Work out the finished part from the listing and answer in its coordinate system (mm). A direction names the side the tool comes from. Round coordinates to 2 decimals unless told otherwise and drop trailing zeros. Loops run counter-clockwise (first coordinate to the right, second up) from the corner with the lowest first, then second, coordinate; pieces in that order, holes last.
```python
from build123d import *

# Parameters (mm, degrees)
SKETCH1_W           = 122
SKETCH1_H           = 30
SKETCH1_R           = 2.2
BOSS_EXTRUDE1_DEPTH = 3
SKETCH2_W           = 46
SKETCH2_H           = 86.2
SKETCH2_R           = 1.75
BOSS_EXTRUDE2_DEPTH = 3
BOSS_EXTRUDE3_DEPTH = 3
FILLET1_R           = 10
CHAMFER1_SIZE       = 1.65
SKETCH4_W           = 32
SKETCH4_H           = 16
SKETCH4_R           = 2
BOSS_EXTRUDE4_DEPTH = 3
CHAMFER2_SIZE       = 6


with BuildPart() as part:
    # Sketch1 → Boss-Extrude1 (new body)
    with BuildSketch(Plane.XY):
        Rectangle(SKETCH1_W, SKETCH1_H)
        with Locations((-56, 5)):
            Circle(SKETCH1_R, mode=Mode.SUBTRACT)
        with Locations(Location((-56, -5, 0), (0, 0, 180))):
            Circle(SKETCH1_R, mode=Mode.SUBTRACT)
        with Locations((56, -5)):
            Circle(SKETCH1_R, mode=Mode.SUBTRACT)
        with Locations(Location((56, 5, 0), (0, 0, 180))):
            Circle(SKETCH1_R, mode=Mode.SUBTRACT)
    extrude(amount=BOSS_EXTRUDE1_DEPTH)

    # Sketch2 → Boss-Extrude2 (add)
    with BuildSketch(Plane.XY.offset(3)):
        with Locations((0, 58.1)):
            Rectangle(SKETCH2_W, SKETCH2_H)
        with Locations((0, 17.3)):
            Circle(SKETCH2_R, mode=Mode.SUBTRACT)
        with Locations((10, 54.9)):
            Circle(SKETCH2_R, mode=Mode.SUBTRACT)
        with Locations((0, 31.2)):
            Circle(SKETCH2_R, mode=Mode.SUBTRACT)
        with Locations(Location((-10, 54.9, 0), (0, 0, 180))):
            Circle(SKETCH2_R, mode=Mode.SUBTRACT)
    extrude(amount=-BOSS_EXTRUDE2_DEPTH)

    # Sketch3 → Boss-Extrude3 (add)
    with BuildSketch(Plane.XY.offset(3)):
        Polygon((-47, 15), (-23, 39), (-23, 15), align=None)
        Polygon((23, 39), (23, 15), (47, 15), align=None)
    extrude(amount=-BOSS_EXTRUDE3_DEPTH)

    # Fillet1
    fillet1_edges = [part.edges().sort_by_distance(p)[0] for p in [
        (-47, 15, 1.5),
        (-23, 39, 1.5),
        (23, 39, 1.5),
        (47, 15, 1.5),
    ]]
    fillet(fillet1_edges, radius=FILLET1_R)

    # Chamfer1
    chamfer1_edges = [part.edges().sort_by_distance(p)[0] for p in [
        (-1.75, 17.3, 3),
        (8.25, 54.9, 3),
        (-1.75, 31.2, 3),
        (-8.25, 54.9, 3),
    ]]
    chamfer(chamfer1_edges, length=CHAMFER1_SIZE)

    # Sketch4 → Boss-Extrude4 (add)
    with BuildSketch(Plane(origin=(23, 0, 0), x_dir=(0, 0, -1), z_dir=(1, 0, 0))):
        with Locations((13, 93.2)):
            Rectangle(SKETCH4_W, SKETCH4_H)
        with Locations(Location((23, 93.2, 0), (0, 0, 90))):
            Circle(SKETCH4_R, mode=Mode.SUBTRACT)
        with Locations(Location((6, 93.2, 0), (0, 0, 270))):
            Circle(SKETCH4_R, mode=Mode.SUBTRACT)
    boss_extrude4 = extrude(amount=-BOSS_EXTRUDE4_DEPTH)

    # Mirror1: Boss-Extrude4 across plane
    add(boss_extrude4.mirror(Plane(origin=(0, 0, 0), x_dir=(0, 0, 1), z_dir=(1, 0, 0))))

    # Chamfer2
    chamfer2_edges = [part.edges().sort_by_distance(p)[0] for p in [
        (21.5, 85.2, 0),
        (-21.5, 85.2, 0),
    ]]
    chamfer(chamfer2_edges, length=CHAMFER2_SIZE)


solid = part.part
```
1. Given pin 1 (1.5 mm diameter, centred on x = 21.5, z = -15.5, fed in from -Y); pin 2 (4 mm diameter, centred on x = -56, y = 5, fed in from -Z); pin 3 (6.5 mm diameter, centred on y = 87.5, z = -18.5, fed in from +X); pin 4 (1.5 mm diameter, centred on x = -54.5, z = 1, fed in from +Y), each flat-ended and moving along its own axis, determine where each tip first touches the part or whether it passes through.
Answer key:
pin 1: stops at y = 85.2
pin 2: passes through
pin 3: stops at x = 23
pin 4: stops at y = 15
2. Find section B-B (y = 31.2). Write down the section's boundary in (x, z).
Answer key:
outline: (-30.8, 0) - (-1.75, 0) - (-1.75, 1.35) - (-3.4, 3) - (-30.8, 3) - close; (1.75, 0) - (30.8, 0) - (30.8, 3) - (3.4, 3) - (1.75, 1.35) - close
3. Find section A-A (z = -11). Write down the section's boundary in (x, y), then the cut area to 3 significant figures.
Answer key:
outline: (-23, 85.2) - (-20, 85.2) - (-20, 101.2) - (-23, 101.2) - close; (20, 85.2) - (23, 85.2) - (23, 101.2) - (20, 101.2) - close
area: 96.0 mm2
4. Find section C-C (x = 10). Write down the section's boundary in (y, z), then the cut area to 3 significant figures.
Answer key:
outline: (-15, 0) - (53.15, 0) - (53.15, 1.35) - (51.5, 3) - (-15, 3) - close; (56.65, 0) - (101.2, 0) - (101.2, 3) - (58.3, 3) - (56.65, 1.35) - close
area: 335 mm2
5. Which of the six approach directions +Z, -Z, +X, -X, +Y, -Y give full straight-line access (tool end or side, diameter ignored) to faces 4 (the face through (56, 15, 1)), 5 (the face through (-10.81, 56.45, 0.68)), 6 (the face through (-22, 85.2, -17))?
Answer key:
face 4: +Z, -Z, +X, +Y
face 5: +Z, -Z
face 6: -Z, +X, -X, -Y
6. Determine the mould class of faces 1 (the face through (-20, 93, -14)), 2 (the face through (35, 27, 2)), 3 (the face through (0.9, 32.7, 0.7)) for opening direction Y: +Y half, -Y half, draft (parallel to the pull), parting line (faces both ways), or undercut.
Answer key:
face 1: draft
face 2: +Y half
face 3: undercut
7. Consider probe 1 along Y at (x, z) = (0, 0.8); probe 2 along Z at (x, y) = (-22, 93); probe 3 along Y at (x, z) = (-56, 1.25). Determine where each line is inside the solid, lowest interval first.
Answer key:
probe 1: y = -15 to 15.55, 19.05 to 29.45, 32.95 to 101.2
probe 2: z = -29 to -24.99, -21.01 to -7.99, -4.01 to 3
probe 3: y = -15 to -7.2, -2.8 to 2.8, 7.2 to 15
8. Find section D-D (y = -5). Write down the section's boundary in (x, z), then the cut area to 3 significant figures.
Answer key:
outline: (-61, 0) - (-58.2, 0) - (-58.2, 3) - (-61, 3) - close; (-53.8, 0) - (53.8, 0) - (53.8, 3) - (-53.8, 3) - close; (58.2, 0) - (61, 0) - (61, 3) - (58.2, 3) - close
area: 340 mm2
